```python
from build123d import *

# Parameters (mm, degrees)
SKETCH_1_W          = 38.8
SKETCH_1_H          = 10.1
EXTRUDE_1_DEPTH     = 60
SKETCH_2_R          = 5
CUT_EXTRUDE_1_DEPTH = 60
SKETCH_3_R          = 2.15
CUT_EXTRUDE_2_DEPTH = 64.862117096


with BuildPart() as part:
    # 草图1 → 凸台-拉伸1 (new body)
    with BuildSketch(Plane(origin=(0, 0, 0), x_dir=(1, 0, 0), z_dir=(0, 1, 0))):
        with Locations((0, 5.05)):
            Rectangle(SKETCH_1_W, SKETCH_1_H)
    extrude(amount=EXTRUDE_1_DEPTH)

    # 草图2 → 切除-拉伸1 (cut)
    with BuildSketch(Plane(origin=(0, 60, 0), x_dir=(1, 0, 0), z_dir=(0, 1, 0))):
        with Locations((0, -0.5)):
            Circle(SKETCH_2_R)
    extrude(amount=-CUT_EXTRUDE_1_DEPTH, mode=Mode.SUBTRACT)

    # 草图3 → 切除-拉伸2 (cut, through all)
    with BuildSketch(Plane(origin=(0, 0, -10.1), x_dir=(-1, 0, 0), z_dir=(0, 0, -1))):
        with Locations((-11.4, 52.5)):
            Circle(SKETCH_3_R)
        with Locations((-11.4, 37.5)):
            Circle(SKETCH_3_R)
        with Locations((-11.4, 22.5)):
            Circle(SKETCH_3_R)
        with Locations((-11.4, 7.5)):
            Circle(SKETCH_3_R)
        with Locations((11.98, 52.5)):
            Circle(SKETCH_3_R)
        with Locations((11.98, 37.5)):
            Circle(SKETCH_3_R)
        with Locations((11.98, 22.5)):
            Circle(SKETCH_3_R)
        with Locations((11.98, 7.5)):
            Circle(SKETCH_3_R)
    extrude(amount=-CUT_EXTRUDE_2_DEPTH, mode=Mode.SUBTRACT)


solid = part.part
```
Geometry check sheet. Reference: the model listing, model coordinates, mm. Coordinates: 2 decimals unless noted, no trailing zeros. Order: outer loops, then holes, each group sorted by start corner. A loop starts at its lowest first (then second) coordinate and runs counter-clockwise, first axis right, second up. Notation, with made-up numbers: M 59.5,78.5 L 79.5,78.5 A19 cw 79.5,101.5 Z; hole C 76.5,-22.5 d4. An arc over 180 degrees is marked long. Answer as a JSON object with one key per item and string values.
Q1. Depth check by flat-ended pin: pin 1 Ø3.5 at (x, y) = (11.4, 22.5) entering from -Z; pin 2 Ø5 at (x, y) = (-11.98, 52.5) entering from -Z; pin 3 Ø3 at (x, y) = (1.5, 23.5) entering from +Z. Enter the tip coordinate at first touch or a pass-through.
Results are:
{"pin 1": "passes through", "pin 2": "stops at z = -10.1", "pin 3": "stops at z = -3.5"}
Q2. Cross-section at B-B on y = 52.5. Record the cut outline in (x, z).
Results are:
{"outline": "M -19.4,-10.1 L -14.13,-10.1 L -14.13,0 L -19.4,0 Z; M -9.83,-10.1 L 9.25,-10.1 L 9.25,0 L 4.97,0 A5 cw -4.97,0 L -9.83,0 Z; M 13.55,-10.1 L 19.4,-10.1 L 19.4,0 L 13.55,0 Z"}
Q3. Scan lines: line 1 (Y direction, x = -11.98, z = -7); line 2 (X direction, y = 21, z = -0.5); line 3 (Y direction, x = 9.5, z = -1.75). Record each from-to range of solid material in increasing order.
Results are:
{"line 1": "y = 0 to 5.35, 9.65 to 20.35, 24.65 to 35.35, 39.65 to 50.35, 54.65 to 60", "line 2": "x = -19.4 to -13.52, -10.44 to -4.9, 4.9 to 9.86, 12.94 to 19.4", "line 3": "y = 0 to 6.49, 8.51 to 21.49, 23.51 to 36.49, 38.51 to 51.49, 53.51 to 60"}
Q4. Cross-section at C-C on z = -2. Give the number of separate pieces and of enclosed holes in the cut face, and give its area (3 significant figures).
Results are:
{"separate pieces": "2", "enclosed holes": "8", "area": "1,690 mm²"}
Q5. Release check for a two-part mould opening along Y. For faces 1 (the cylindrical face through (-9.83, 52.59, -5.12)), 2 (the flat face through (0, 0, -5)), 3 (the cylindrical face through (11.68, 9.63, -5.12)), 4 (the flat face through (19.4, 30, -5)) record: released by +Y, released by -Y, zero draft, split by the parting line, or undercut.
Results are:
{"face 1": "undercut", "face 2": "released by -Y", "face 3": "undercut", "face 4": "zero draft"}
Q6. Cross-section at A-A on x = 11.4. Record the cut outline in (y, z).
Results are:
{"outline": "M 0,-10.1 L 5.35,-10.1 L 5.35,0 L 0,0 Z; M 9.65,-10.1 L 20.35,-10.1 L 20.35,0 L 9.65,0 Z; M 24.65,-10.1 L 35.35,-10.1 L 35.35,0 L 24.65,0 Z; M 39.65,-10.1 L 50.35,-10.1 L 50.35,0 L 39.65,0 Z; M 54.65,-10.1 L 60,-10.1 L 60,0 L 54.65,0 Z"}
